Geometry check sheet. Reference: the model listing, model coordinates, mm. Face numbers are marked on the shaded views. A direction names the side the tool comes from. Give positions to 0.01 mm unless a question says otherwise; leave off trailing zeros. Order: outer loops, then holes, each group sorted by start corner. A loop starts at its lowest first (then second) coordinate and runs counter-clockwise, first axis right, second up.
from build123d import *

# Parameters (mm, degrees)
PAD_DEPTH       = 5
FILLET_R        = 1
FILLET001_R     = 1
FILLET002_R     = 1
SKETCH001_R     = 1.75
PAD001_DEPTH    = 2
SKETCH002_W     = 61.2
SKETCH002_H     = 76.2
PAD002_DEPTH    = 2
PAD003_DEPTH    = 55
SKETCH004_W     = 35
SKETCH004_H     = 25
SKETCH004_W_2   = 14.2
SKETCH004_H_2   = 19
SKETCH004_W_3   = 51.2
SKETCH004_H_3   = 20
POCKET_DEPTH    = 2
SKETCH005_W     = 14.2
SKETCH005_H     = 19
SKETCH005_W_2   = 51.2
SKETCH005_H_2   = 20
POCKET001_DEPTH = 2
SKETCH006_W     = 66.2
SKETCH006_H     = 19
SKETCH006_H_2   = 20
POCKET002_DEPTH = 2
SKETCH007_W     = 24.2
SKETCH007_H     = 10
PAD004_DEPTH    = 2
SKETCH008_W     = 2
SKETCH008_H     = 10
PAD005_DEPTH    = 25
PAD006_DEPTH    = 2
SKETCH010_W     = 2
SKETCH010_H     = 4
PAD007_DEPTH    = 2
SKETCH011_W     = 6
SKETCH011_H     = 6
SKETCH011_R     = 1.25
PAD008_DEPTH    = 4


with BuildPart() as part:
    # Sketch → Pad (new body)
    with BuildSketch(Plane.XY):
        Polygon((28.537386, 0), (-14.268693, 24.714102), (-14.268693, -24.714102), align=None)
        Polygon((24.537386, 0), (-12.268693, 21.25), (-12.268693, -21.25), align=None, mode=Mode.SUBTRACT)
    extrude(amount=PAD_DEPTH)

    # Fillet
    fillet_edges = [part.edges().sort_by_distance(p)[0] for p in [
        (-14.268693, -24.714102, 2.5),
    ]]
    fillet(fillet_edges, radius=FILLET_R)

    # Fillet001
    fillet001_edges = [part.edges().sort_by_distance(p)[0] for p in [
        (28.537386, 0, 2.5),
    ]]
    fillet(fillet001_edges, radius=FILLET001_R)

    # Fillet002
    fillet002_edges = [part.edges().sort_by_distance(p)[0] for p in [
        (-14.268693, 24.714102, 2.5),
    ]]
    fillet(fillet002_edges, radius=FILLET002_R)

    # Sketch001 (on Face1 of Fillet002) → Pad001 (join)
    with BuildSketch(Plane(origin=(0, 0, 0), x_dir=(1, 0, 0), z_dir=(0, 0, -1))):
        Polygon((24.537386, 0), (-12.268693, 21.25), (-12.268693, -21.25), align=None)
        with Locations((4.134347, 7.160898)):
            Circle(SKETCH001_R, mode=Mode.SUBTRACT)
        with Locations((4.134347, -7.160898)):
            Circle(SKETCH001_R, mode=Mode.SUBTRACT)
        with Locations((-8.268693, 0)):
            Circle(SKETCH001_R, mode=Mode.SUBTRACT)
        Polygon((8.537386, 0), (-4.268693, 7.393594), (-4.268693, -7.393594), align=None, mode=Mode.SUBTRACT)
    extrude(amount=-PAD001_DEPTH)

    # Sketch002 (on Face9 of Pad001) → Pad002 (join)
    with BuildSketch(Plane.XY.offset(5)):
        with Locations((-1.062614, -0.09)):
            Rectangle(SKETCH002_W, SKETCH002_H)
        Polygon((-12.268693, 21.25), (-12.268693, -21.25), (24.537386, 0), align=None, mode=Mode.SUBTRACT)
    extrude(amount=PAD002_DEPTH)

    # Sketch003 (on Face21 of Pad002) → Pad003 (join)
    with BuildSketch(Plane.XY.offset(7)):
        Polygon((-31.662614, 38.01), (29.537386, 38.01), (29.537386, -38.19), (-31.662614, -38.19), (-31.662614, -36.19), (27.537386, -36.19), (27.537386, 36.01), (-31.662614, 36.01), align=None)
    extrude(amount=PAD003_DEPTH)

    # Sketch004 (on Face26 of Pad003) → Pocket (cut)
    with BuildSketch(Plane.XZ.offset(38.19)):
        with Locations((10.037386, 19.5)):
            Rectangle(SKETCH004_W, SKETCH004_H)
        with Locations((-19.562614, 19.5)):
            Rectangle(SKETCH004_W_2, SKETCH004_H_2)
        with Locations((-1.062614, 47)):
            Rectangle(SKETCH004_W_3, SKETCH004_H_3)
    extrude(amount=-POCKET_DEPTH, mode=Mode.SUBTRACT)

    # Sketch005 (on Face21 of Pocket) → Pocket001 (cut)
    with BuildSketch(Plane(origin=(0, 38.01, 0), x_dir=(-1, 0, 0), z_dir=(0, 1, 0))):
        Polygon((-24.537386, 32), (-12.537386, 32), (-12.537386, 34), (7.462614, 34), (7.462614, 32), (7.462614, 10), (-24.537386, 10), align=None)
        with Locations((19.562614, 19.5)):
            Rectangle(SKETCH005_W, SKETCH005_H)
        with Locations((1.062614, 47)):
            Rectangle(SKETCH005_W_2, SKETCH005_H_2)
    extrude(amount=-POCKET001_DEPTH, mode=Mode.SUBTRACT)

    # Sketch006 (on Face25 of Pocket001) → Pocket002 (cut)
    with BuildSketch(Plane.YZ.offset(29.537386)):
        with Locations((-0.09, 19.5)):
            Rectangle(SKETCH006_W, SKETCH006_H)
        with Locations((-0.09, 47)):
            Rectangle(SKETCH006_W, SKETCH006_H_2)
    extrude(amount=-POCKET002_DEPTH, mode=Mode.SUBTRACT)

    # Sketch007 (on Face62 of Pocket002) → Pad004 (join)
    with BuildSketch(Plane(origin=(0, 0, 32), x_dir=(1, 0, 0), z_dir=(0, 0, -1))):
        Polygon((-31.662614, 36.19), (-31.662614, 26.19), (17.537386, 26.19), (17.537386, -26.01), (12.537386, -26.01), (12.537386, -36.01), (27.537386, -36.01), (27.537386, 36.19), align=None)
        with Locations((-19.562614, -31.01)):
            Rectangle(SKETCH007_W, SKETCH007_H)
    extrude(amount=-PAD004_DEPTH)

    # Sketch008 (on Face79 of Pad004) → Pad005 (join)
    with BuildSketch(Plane(origin=(0, 0, 32), x_dir=(1, 0, 0), z_dir=(0, 0, -1))):
        with Locations((-8.462614, 31.19)):
            Rectangle(SKETCH008_W, SKETCH008_H)
        with Locations((-8.462614, -31.01)):
            Rectangle(SKETCH008_W, SKETCH008_H)
    extrude(amount=PAD005_DEPTH)

    # Sketch009 (on Face31 of Pad005) → Pad006 (join)
    with BuildSketch(Plane.XY.offset(62)):
        Polygon((-31.662614, 36.01), (27.537386, 36.01), (27.537386, -36.19), (-31.662614, -36.19), (-31.662614, -32.19), (-27.662614, -32.19), (-27.662614, -34.19), (25.537386, -34.19), (25.537386, 34.01), (-27.662614, 34.01), (-27.662614, 32.01), (-31.662614, 32.01), align=None)
    extrude(amount=-PAD006_DEPTH)

    # Sketch010 (on Face92 of Pad006) → Pad007 (join)
    with BuildSketch(Plane(origin=(0, 0, 60), x_dir=(1, 0, 0), z_dir=(0, 0, -1))):
        with Locations((-30.662614, 34.19)):
            Rectangle(SKETCH010_W, SKETCH010_H)
        with Locations((-30.662614, -34.01)):
            Rectangle(SKETCH010_W, SKETCH010_H)
    extrude(amount=PAD007_DEPTH)

    # Sketch011 (on Face17 of Pad007) → Pad008 (join)
    with BuildSketch(Plane(origin=(-31.662614, 0, 0), x_dir=(0, -1, 0), z_dir=(-1, 0, 0))):
        with Locations((-8.81, 2)):
            Rectangle(SKETCH011_W, SKETCH011_H)
        with Locations((-8.81, 2)):
            Circle(SKETCH011_R, mode=Mode.SUBTRACT)
        with Locations((31.19, 2)):
            Rectangle(SKETCH011_W, SKETCH011_H)
        with Locations((31.19, 2)):
            Circle(SKETCH011_R, mode=Mode.SUBTRACT)
    extrude(amount=-PAD008_DEPTH)


solid = part.part
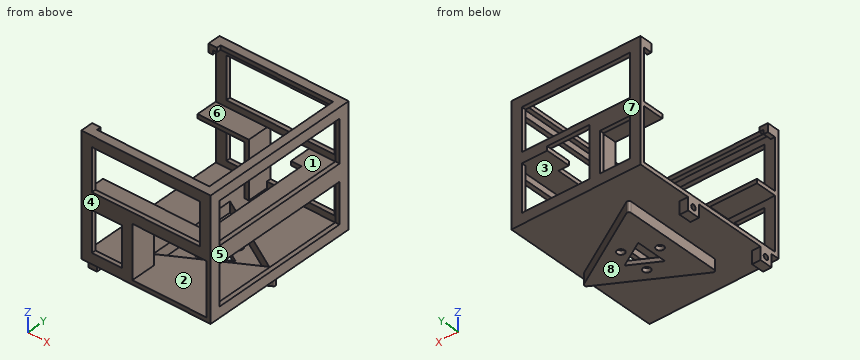
Item 1: Sectioned sample at C-C (z = 30). Enter the section's corners in (x, y).
Reported:
outline: (-31.66, -38.19) - (-7.46, -38.19) - (-7.46, -26.19) - (-9.46, -26.19) - (-9.46, -36.19) - (-31.66, -36.19) - close; (-31.66, 36.01) - (-9.46, 36.01) - (-9.46, 26.01) - (-7.46, 26.01) - (-7.46, 38.01) - (-31.66, 38.01) - close; (24.54, 36.01) - (27.54, 36.01) - (27.54, -38.19) - (29.54, -38.19) - (29.54, 38.01) - (24.54, 38.01) - close
Item 2: Sectioned sample at D-D (z = 8.5). Enter the section's corners in (x, y).
Reported:
outline: (-31.66, -38.19) - (-7.46, -38.19) - (-7.46, -26.19) - (-9.46, -26.19) - (-9.46, -36.19) - (-31.66, -36.19) - close; (-31.66, 36.01) - (-9.46, 36.01) - (-9.46, 26.01) - (-7.46, 26.01) - (-7.46, 36.01) - (27.54, 36.01) - (27.54, -38.19) - (29.54, -38.19) - (29.54, 38.01) - (-31.66, 38.01) - close
Item 3: Set-up check for the marked faces 1, 2, 3, 4 and 5: record each of +Z, -Z, +X, -X, +Y, -Y from which the full face is reachable in a straight line by a thin tool's end or side.
Reported:
face 1: -X
face 2: none
face 3: -Y
face 4: +Z, -Z, +X, -X, -Y
face 5: +Z, -Z, +X, +Y, -Y
Item 4: Scan lines: L1, parallel to Z at x = -30.45, y = -31.19; L2, parallel to Y at x = -3, z = 35.5; L3, parallel to Z at x = 23.5, y = 7. Record each from-to range of solid material in increasing order.
Reported:
L1: z = -1 to 0.75, 3.25 to 7, 32 to 34
L2: y = -38.19 to -36.19, 36.01 to 38.01
L3: z = 5 to 7, 32 to 34
Item 5: Draft check along Y on the marked faces 6, 7 and 8. Enter one of: released by +Y, released by -Y, zero draft, split by the parting line, or undercut.
Reported:
face 6: undercut
face 7: released by +Y
face 8: zero draft
Item 6: Gauge pin test, flat ends, axial feed: pin 1 (1.5 mm diameter, centred on x = 19, y = -25, fed in from +Z); pin 2 (0.6 mm diameter, centred on x = 2.5, y = -37.5, fed in from -Z); pin 3 (4.5 mm diameter, centred on x = -29.5, z = 1, fed in from -Y). Record the tip position at first contact, or that the pin passes through.
Reported:
pin 1: stops at z = 34
pin 2: stops at z = 5
pin 3: stops at y = -34.19
Item 7: Sectioned sample at A-A (z = 16). Give the number of separate pieces and of enclosed holes in the cut face, and give its area (3 significant figures).
Reported:
separate pieces: 6
enclosed holes: 0
area: 106 mm2
Item 8: Sectioned sample at B-B (y = 29). Enter the section's corners in (x, z).
Reported:
outline: (-31.66, 5) - (29.54, 5) - (29.54, 10) - (27.54, 10) - (27.54, 7) - (-7.46, 7) - (-7.46, 34) - (-31.66, 34) - (-31.66, 32) - (-9.46, 32) - (-9.46, 7) - (-31.66, 7) - close; (12.54, 32) - (27.54, 32) - (27.54, 29) - (29.54, 29) - (29.54, 37) - (27.54, 37) - (27.54, 34) - (12.54, 34) - close; (25.54, 60) - (27.54, 60) - (27.54, 57) - (29.54, 57) - (29.54, 62) - (25.54, 62) - close
